The listing builds one solid part. Answer for the finished solid, in the listing's coordinates (mm). A direction names the side the tool comes from. Give positions to 0.01 mm unless a question says otherwise; leave off trailing zeros. Write each loop counter-clockwise with the first axis right and the second up, starting at its lowest first coordinate (ties: lowest second). Pieces come first, ordered by that corner, then holes. Notation, with made-up numbers: (-19.5, 53.25) - (5.5, 53.25) arc R15 ccw to (5.5, 62.25) - close; hole circle Ø11 at (31, 54.25). An arc over 180 degrees is marked (long way). One line per question, with ' | ' between items. Start each with the question number.
1. A cutting plane is placed at B-B (y = -22.5). Determine the outline of the cut face in (x, z).
2. Find the intervals of material crossed by L1, parallel to Y at x = 14.5, z = 249.5; L2, parallel to X at y = 9, z = 250.75; L3, parallel to X at y = -26.5, z = 246.75, in increasing order. Write a range as from..to.
3. For faces 1 (the face through (-10.216, 8, 253)), 2 (the face through (5.5, 10, 241)), 3 (the face through (21.11, -1, 247.97)), determine the directions among +Z, -Z, +X, -X, +Y, -Y from which every point of the face is accessible in a straight line to the end or side of a thin tool.
4. A cutting plane is placed at A-A (z = 240). Determine the outline of the cut face in (x, y).
5. A cutting plane is placed at C-C (z = 247). State how many separate pieces and enclosed holes the cut face has, then the cut area to 3 significant figures.
6. The mould has two halves that part along Z. Classify faces 4 (the face through (25, -6, 250)), 5 (the face through (21.159, -7.104, 247.972)), 6 (the face through (0, 9, 241)), 7 (the face through (0, 12, 248.9)): +Z half, -Z half, draft (parallel to the pull), parting line (faces both ways), or undercut.
7. Given P1, Ø1.5, axis at y = 10, z = 244.5, coming from the +X side; P2, Ø5, axis at y = 5.5, z = 253, coming from the +X side; P3, Ø2.5, axis at x = 0, y = 12, coming from the -Z side, each flat-ended and moving along its own axis, determine where each tip first touches the part or whether it passes through.
```python
from build123d import *

# Parameters (mm, degrees)
BOSS_EXTRUDE1_DEPTH      = 13.5
BOSS_EXTRUDE2_DEPTH      = 18.5
BOSS_EXTRUDE3_DEPTH      = 5
SKETCH4_W                = 45.922011884
SKETCH4_H                = 20
BOSS_EXTRUDE4_DEPTH      = 13.5
SKETCH2_R                = 4.25
CUT_EXTRUDE1_DEPTH       = 268.629329099
SKETCH6_R                = 8.05
CUT_EXTRUDE3_DEPTH       = 14
BOSS_EXTRUDE5_DEPTH      = 13.5
CUT_EXTRUDE5_REACH       = 210.1
CUT_EXTRUDE5_END_RADIUS  = 45
SKETCH8_R                = 9
CUT_EXTRUDE6_REACH       = 210.1
SKETCH10_R               = 4
SKETCH11_R               = 8
CUT_EXTRUDE7_DEPTH       = 4
SKETCH18_R               = 11
CUT_EXTRUDE9_DEPTH       = 47
CUT_EXTRUDE11_DEPTH      = 268.629329099
CUT_EXTRUDE11_DEPTH_BACK = 268.629329099
SKETCH20_W               = 45.922011884
SKETCH20_H               = 204.425421037
SKETCH21_W               = 45.922011884
SKETCH21_H               = 10
BOSS_EXTRUDE6_DEPTH      = 16
M5_CLEARANCE_HOLE1_D     = 5.5
CUT_EXTRUDE12_DEPTH      = 5
LPATTERN2_COUNT          = 2
LPATTERN2_PITCH          = 32
LPATTERN2_COPY_1_D       = 5.5
CUT_EXTRUDE13_START      = -4
SKETCH25_R               = 2.75
CUT_EXTRUDE13_DEPTH      = 39.396436099
SKETCH26_W               = 45.922011884
SKETCH26_H               = 10
CUT_EXTRUDE14_DEPTH      = 271.429672547
FILLET1_R                = 5
SKETCH30_W               = 11
SKETCH30_H               = 7
BOSS_EXTRUDE8_DEPTH      = 5
CUT_EXTRUDE15_DEPTH      = 5
FILLET3_R                = 2
BOSS_EXTRUDE9_DEPTH      = 2
BOSS_EXTRUDE10_DEPTH     = 3.75
SKETCH36_W               = 11
SKETCH36_H               = 2.1
CUT_EXTRUDE17_DEPTH      = 2.5
FILLET4_R                = 0.5
BOSS_EXTRUDE11_START     = -10
BOSS_EXTRUDE11_DEPTH     = 10
CUT_EXTRUDE18_DEPTH      = 4
M4_CLEARANCE_HOLE1_D     = 4.5


with BuildPart() as part:
    # Sketch1 → Boss-Extrude1 (new, symmetric)
    with BuildSketch(Plane(origin=(0, 0, 0), x_dir=(1, 0, 0), z_dir=(0, 1, 0))):
        with BuildLine():
            ThreePointArc((17.220754456, -41.574578963), (0, -45), (-17.220754456, -41.574578963))
            Line((-17.220754456, -41.574578963), (-22.961005942, -55.432771951))
            ThreePointArc((-22.961005942, -55.432771951), (0, -60), (22.961005942, -55.432771951))
            Line((22.961005942, -55.432771951), (17.220754456, -41.574578963))
        make_face()
    extrude(amount=BOSS_EXTRUDE1_DEPTH, both=True)

    # Sketch1<3> → Boss-Extrude2 (add, symmetric)
    with BuildSketch(Plane(origin=(0, 0, 0), x_dir=(1, 0, 0), z_dir=(0, 1, 0))):
        with BuildLine():
            ThreePointArc((19.134171618, -46.193976626), (0, -50), (-19.134171618, -46.193976626))
            Line((-19.134171618, -46.193976626), (-21.04758878, -50.813374288))
            ThreePointArc((-21.04758878, -50.813374288), (0, -55), (21.04758878, -50.813374288))
            Line((21.04758878, -50.813374288), (19.134171618, -46.193976626))
        make_face()
    extrude(amount=BOSS_EXTRUDE2_DEPTH, both=True)

    # Sketch3 → Boss-Extrude3 (add, symmetric)
    with BuildSketch(Plane.XZ):
        with BuildLine():
            Line((-22.961005942, 266), (-22.961005942, 55.432771951))
            ThreePointArc((-22.961005942, 55.432771951), (-20.481139434, 56.39612511), (-17.961005942, 57.248600555))
            Line((-17.961005942, 57.248600555), (-17.961005942, 246))
            Line((-17.961005942, 246), (17.961005942, 246))
            Line((17.961005942, 246), (17.961005942, 57.248600555))
            ThreePointArc((17.961005942, 57.248600555), (20.481139434, 56.39612511), (22.961005942, 55.432771951))
            Line((22.961005942, 55.432771951), (22.961005942, 266))
            Line((22.961005942, 266), (-22.961005942, 266))
        make_face()
    extrude(amount=BOSS_EXTRUDE3_DEPTH, both=True)

    # Sketch4 → Boss-Extrude4 (add, symmetric)
    with BuildSketch(Plane(origin=(0, 0, 0), x_dir=(1, 0, 0), z_dir=(0, 1, 0))):
        with Locations((0, -256)):
            Rectangle(SKETCH4_W, SKETCH4_H)
    extrude(amount=BOSS_EXTRUDE4_DEPTH, both=True)

    # Sketch2 → Cut-Extrude1 (cut, through all)
    with BuildSketch(Plane.XY):
        with Locations(Location((0, 0, 0), (0, 0, 180))):
            Circle(SKETCH2_R)
    extrude(amount=CUT_EXTRUDE1_DEPTH, mode=Mode.SUBTRACT)

    # Sketch6 → Cut-Extrude3 (cut)
    with BuildSketch(Plane.XY.offset(266)):
        Circle(SKETCH6_R)
    extrude(amount=-CUT_EXTRUDE3_DEPTH, mode=Mode.SUBTRACT)

    # Sketch9 → Boss-Extrude5 (add, symmetric)
    with BuildSketch(Plane(origin=(0, 0, 0), x_dir=(1, 0, 0), z_dir=(0, 1, 0))):
        with BuildLine():
            Line((-22.961005942, -55.432771951), (-22.961005942, -68))
            Line((-22.961005942, -68), (22.961005942, -68))
            Line((22.961005942, -68), (22.961005942, -55.432771951))
            ThreePointArc((22.961005942, -55.432771951), (0, -60), (-22.961005942, -55.432771951))
        make_face()
    extrude(amount=BOSS_EXTRUDE5_DEPTH, both=True)

    # Cut-Extrude5: up to this cylinder (the profile starts outside it)
    cut_extrude5_end = Plane(origin=(0, 0, 0), z_dir=(0, -1, 0)) * Cylinder(CUT_EXTRUDE5_END_RADIUS, 511.2, mode=Mode.PRIVATE)
    # Sketch8 → Cut-Extrude5 (cut, up to the surface)
    with BuildSketch(Plane.XY.offset(60), mode=Mode.PRIVATE) as cut_extrude5_sk1:
        Circle(SKETCH8_R)
    cut_extrude5_tool1 = extrude(cut_extrude5_sk1.sketch, amount=-CUT_EXTRUDE5_REACH, mode=Mode.PRIVATE) - cut_extrude5_end
    add(cut_extrude5_tool1.solids().sort_by_distance((0, 0, 60))[0], mode=Mode.SUBTRACT)

    # Sketch10 → Cut-Extrude6 (cut, up to next)
    with BuildSketch(Plane.XY.offset(60), mode=Mode.PRIVATE) as cut_extrude6_sk1:
        with Locations(Location((0, 0, 0), (0, 0, 180))):
            Circle(SKETCH10_R)
    cut_extrude6_tool1 = extrude(cut_extrude6_sk1.sketch, amount=CUT_EXTRUDE6_REACH, mode=Mode.PRIVATE) & part.part
    add(cut_extrude6_tool1.solids().sort_by_distance((0, 0, 60))[0], mode=Mode.SUBTRACT)

    # Sketch11 → Cut-Extrude7 (cut)
    with BuildSketch(Plane.XY.offset(68)):
        Circle(SKETCH11_R)
    extrude(amount=-CUT_EXTRUDE7_DEPTH, mode=Mode.SUBTRACT)

    # Sketch18 → Cut-Extrude9 (cut)
    with BuildSketch(Plane.XY):
        with Locations(Location((0, 0, 0), (0, 0, 180))):
            Circle(SKETCH18_R)
    extrude(amount=CUT_EXTRUDE9_DEPTH, mode=Mode.SUBTRACT)

    # Sketch20 → Cut-Extrude11 (cut, two sides: drawn at the far end of the back side and taken through both)
    with BuildSketch(Plane(origin=(0, 0, 0), x_dir=(1, 0, 0), z_dir=(0, 1, 0)).offset(-CUT_EXTRUDE11_DEPTH_BACK)):
        with Locations((0, -143.787289482)):
            Rectangle(SKETCH20_W, SKETCH20_H)
    extrude(amount=CUT_EXTRUDE11_DEPTH + CUT_EXTRUDE11_DEPTH_BACK, mode=Mode.SUBTRACT)

    # Sketch21 → Boss-Extrude6 (add)
    with BuildSketch(Plane.XZ.offset(13.5)):
        with Locations((0, 251)):
            Rectangle(SKETCH21_W, SKETCH21_H)
    extrude(amount=BOSS_EXTRUDE6_DEPTH)

    # M5 Clearance Hole1 (through all)
    with Locations(Plane(origin=(0, 0, 246), x_dir=(-1, 0, 0), z_dir=(0, 0, -1))):
        with Locations((-14.26606865, -24)):
            m5_clearance_hole1 = Hole(M5_CLEARANCE_HOLE1_D / 2)

    # Sketch24 → Cut-Extrude12 (cut)
    with BuildSketch(Plane.XY.offset(256)):
        Polygon((18.94260583, -24), (16.60433724, -19.95), (11.92780006, -19.95), (9.58953147, -24), (11.92780006, -28.05), (16.60433724, -28.05), align=None)
    cut_extrude12 = extrude(amount=-CUT_EXTRUDE12_DEPTH, mode=Mode.SUBTRACT)

    # Mirror1: M5 Clearance Hole1 across plane
    add(m5_clearance_hole1.mirror(Plane(origin=(0, 0, 0), x_dir=(0, 0, 1), z_dir=(1, 0, 0))), mode=Mode.SUBTRACT)

    # Mirror2: Cut-Extrude12 across plane
    add(cut_extrude12.mirror(Plane(origin=(0, 0, 0), x_dir=(0, 0, 1), z_dir=(1, 0, 0))), mode=Mode.SUBTRACT)

    # LPattern2: M5 Clearance Hole1 ×2
    with Locations(*[(0, i * LPATTERN2_PITCH, 0) for i in range(1, LPATTERN2_COUNT)]):
        add(m5_clearance_hole1, mode=Mode.SUBTRACT)

    # LPattern2 copy 1 (through all)
    with Locations(Plane(origin=(0, 32, 246), x_dir=(1, 0, 0), z_dir=(0, 0, -1))):
        with Locations((-14.26606865, 24)):
            Hole(LPATTERN2_COPY_1_D / 2)

    # Sketch25 → Cut-Extrude13 (cut, through all)
    # profile 1 of 2: a face of its own
    with BuildSketch(Plane(origin=(0, 0, 246), x_dir=(-1, 0, 0), z_dir=(0, 0, -1)).offset(CUT_EXTRUDE13_START)):
        Polygon((-10.21606865, 10.33826859), (-14.26606865, 12.67653718), (-18.31606865, 10.33826859), (-18.31606865, 5.66173141), (-14.26606865, 3.32346282), (-10.21606865, 5.66173141), align=None)
        with Locations((-14.26606865, 8)):
            Circle(SKETCH25_R, mode=Mode.SUBTRACT)
    # profile 2 of 2: a face of its own
    with BuildSketch(Plane(origin=(0, 0, 246), x_dir=(-1, 0, 0), z_dir=(0, 0, -1)).offset(CUT_EXTRUDE13_START)):
        with Locations((-14.26606865, 8)):
            Circle(SKETCH25_R)
    cut_extrude13 = extrude(amount=-CUT_EXTRUDE13_DEPTH, mode=Mode.SUBTRACT)

    # Mirror3: Cut-Extrude13 across plane
    add(cut_extrude13.mirror(Plane(origin=(0, 0, 0), x_dir=(0, 0, 1), z_dir=(1, 0, 0))), mode=Mode.SUBTRACT)

    # Sketch26 → Cut-Extrude14 (cut, through all)
    with BuildSketch(Plane(origin=(0, 13.5, 0), x_dir=(1, 0, 0), z_dir=(0, 1, 0))):
        with Locations((0, -261)):
            Rectangle(SKETCH26_W, SKETCH26_H)
    extrude(amount=-CUT_EXTRUDE14_DEPTH, mode=Mode.SUBTRACT)

    # Fillet1
    fillet1_edges = [part.edges().sort_by_distance(p)[0] for p in [
        (-22.961005942, -29.5, 251),
        (22.961005942, -29.5, 251),
        (22.961005942, 13.5, 251),
        (-22.961005942, 13.5, 251),
    ]]
    fillet(fillet1_edges, radius=FILLET1_R)

    # Sketch30 → Boss-Extrude8 (add)
    with BuildSketch(Plane(origin=(0, 0, 246), x_dir=(-1, 0, 0), z_dir=(0, 0, -1))):
        with Locations((0, 10)):
            Rectangle(SKETCH30_W, SKETCH30_H)
    extrude(amount=BOSS_EXTRUDE8_DEPTH)

    # Sketch31 → Cut-Extrude15 (cut)
    with BuildSketch(Plane(origin=(0, 13.5, 0), x_dir=(1, 0, 0), z_dir=(0, 1, 0))):
        Polygon((3.735, -241), (3.735, -248), (3.235, -248), (3.235, -245.2), (-3.235, -245.2), (-3.235, -248), (-3.735, -248), (-3.735, -241), align=None)
    extrude(amount=-CUT_EXTRUDE15_DEPTH, mode=Mode.SUBTRACT)

    # Fillet3
    fillet3_edges = [part.edges().sort_by_distance(p)[0] for p in [
        (-5.5, 10, 246),
        (5.5, 10, 246),
        (0, 6.5, 246),
    ]]
    fillet(fillet3_edges, radius=FILLET3_R)

    # Sketch32 → Boss-Extrude9 (add)
    with BuildSketch(Plane(origin=(0, 0, 241), x_dir=(-1, 0, 0), z_dir=(0, 0, -1))):
        Polygon((3.735, 13.5), (3.735, 8.5), (-3.735, 8.5), (-3.735, 13.5), (-5.5, 13.5), (-5.5, 6.5), (5.5, 6.5), (5.5, 13.5), align=None)
        with BuildLine():
            ThreePointArc((1.75, 11.5), (0, 9.75), (-1.75, 11.5))
            Line((-1.75, 11.5), (-1.75, 13.5))
            Line((-1.75, 13.5), (-3.735, 13.5))
            Line((-3.735, 13.5), (-3.735, 8.5))
            Line((-3.735, 8.5), (3.735, 8.5))
            Line((3.735, 8.5), (3.735, 13.5))
            Line((3.735, 13.5), (1.75, 13.5))
            Line((1.75, 13.5), (1.75, 11.5))
        make_face()
    extrude(amount=BOSS_EXTRUDE9_DEPTH)

    # Sketch34 → Boss-Extrude10 (add)
    with BuildSketch(Plane.ZY.offset(5.5)):
        with BuildLine():
            Line((239, 13.5), (239, 11.5))
            ThreePointArc((239, 11.5), (238, 12.5), (239, 13.5))
        make_face()
    boss_extrude10 = extrude(amount=-BOSS_EXTRUDE10_DEPTH)

    # Mirror5: Boss-Extrude10 across plane
    add(boss_extrude10.mirror(Plane(origin=(0, 0, 0), x_dir=(0, 0, 1), z_dir=(1, 0, 0))))

    # Sketch36 → Cut-Extrude17 (cut)
    with BuildSketch(Plane(origin=(0, 13.5, 0), x_dir=(1, 0, 0), z_dir=(0, 1, 0))):
        with Locations((0, -249.95)):
            Rectangle(SKETCH36_W, SKETCH36_H)
    extrude(amount=-CUT_EXTRUDE17_DEPTH, mode=Mode.SUBTRACT)

    # Fillet4
    fillet4_edges = [part.edges().sort_by_distance(p)[0] for p in [
        (0, 13.5, 248.9),
    ]]
    fillet(fillet4_edges, radius=FILLET4_R)

    # Sketch38 → Boss-Extrude11 (add)
    with BuildSketch(Plane.XY.offset(256).offset(BOSS_EXTRUDE11_START)):
        with BuildLine():
            Line((23.938669324, 1.871526387), (22.961005942, 2.04391482))
            Line((22.961005942, 2.04391482), (22.961005942, -10.036976376))
            ThreePointArc((22.961005942, -10.036976376), (28.876661693, -4.528255996), (23.938669324, 1.871526387))
        make_face()
        with BuildLine():
            ThreePointArc((-22.961005942, 8.5), (-22.900298084, 9.276783841), (-22.719648688, 10.034704928))
            ThreePointArc((-22.719648688, 10.034704928), (-28.86557724, 4.648435983), (-23.938669324, -1.871526387))
            Line((-23.938669324, -1.871526387), (-22.961005942, -2.04391482))
            Line((-22.961005942, -2.04391482), (-22.961005942, 8.5))
        make_face()
    extrude(amount=BOSS_EXTRUDE11_DEPTH)

    # Sketch39 → Cut-Extrude18 (cut)
    with BuildSketch(Plane(origin=(0, 0, 246), x_dir=(-1, 0, 0), z_dir=(0, 0, -1))):
        Polygon((-22.896780258, -8.107639529), (-19.371780258, -6.07247983), (-19.371780258, -2.002160432), (-22.896780258, 0.032999267), (-26.421780258, -2.002160432), (-26.421780258, -6.07247983), align=None)
        Polygon((18.894288787, 3.29734579), (21.536371099, 0.201073668), (25.53886257, 0.941048009), (26.899271729, 4.777294471), (24.257189416, 7.873566593), (20.254697945, 7.133592253), align=None)
    extrude(amount=-CUT_EXTRUDE18_DEPTH, mode=Mode.SUBTRACT)

    # M4 Clearance Hole1 (through all)
    with Locations(Plane.XY.offset(256)):
        with Locations((-22.896780258, 4.037320131), (22.896780258, -4.037320131)):
            Hole(M4_CLEARANCE_HOLE1_D / 2)


solid = part.part
```
Determined:
1) outline: (-22.96, 246) - (-16.57, 246) - (-16.57, 251) - (-18.08, 251) - (-18.08, 256) - (-22.96, 256) - close; (-11.96, 246) - (11.96, 246) - (11.96, 251) - (10.46, 251) - (10.46, 256) - (-10.46, 256) - (-10.46, 251) - (-11.96, 251) - close; (16.57, 246) - (22.96, 246) - (22.96, 256) - (18.08, 256) - (18.08, 251) - (16.57, 251) - close
2) L1: -29.5..-26.74, -21.26..5.26, 10.74..13.5 | L2: -26.27..-18.32, -10.22..10.22, 18.32..22.94 | L3: -22.54..-15.41, -13.12..13.12, 15.41..22.54
3) face 1: +Z | face 2: -Z, +X, +Y, -Y | face 3: -Z
4) outline: (-5.5, 6.5) - (5.5, 6.5) - (5.5, 13.5) - (1.75, 13.5) - (1.75, 11.5) arc R1.75 cw to (-1.75, 11.5) - (-1.75, 13.5) - (-5.5, 13.5) - close
5) separate pieces: 1 | enclosed holes: 7 | area: 1,820 mm2
6) face 4: -Z half | face 5: draft | face 6: undercut | face 7: undercut
7) P1: x = 5.94 | P2: x = 22.96 | P3: z = 245.2
